Autodesk Fusion 360 part; units mm, degrees
sketch "Sketch1" plane through (0, 0, 0) normal (0, 0, 1) x (1, 0, 0)
  circle A0 centre (0, 0) radius 23.05
  line L0 (4.05, 4.05) -> (-4.05, 4.05) construction
  line L1 (-4.05, 4.05) -> (-4.05, -4.05) construction
  line L2 (-4.05, -4.05) -> (4.05, -4.05) construction
  line L3 (4.05, -4.05) -> (4.05, 4.05) construction
  line L4 (4.05, 4.05) -> (-4.05, -4.05) construction
  line L5 (-4.05, 4.05) -> (4.05, -4.05) construction
  circle A1 centre (0, 0) radius 1.95
  circle A2 centre (0, 0) radius 12
  line L6 (0, 0) -> (-9, -21.2203)
  line L7 (0, 0) -> (9, -21.2203)
  arc A3 (7.0767, -16.6855) -> (-7.0767, -16.6855) centre (0, -19.6868) ccw
  dimension "d1" = 46.1
  dimension "d2" = 8.1
  dimension "d3" = 8.1
  dimension "d4" = 3.9
  dimension "d5" = 24
  dimension "d19" = 18
  dimension "d20" = 9
extrude "Extrude1" add sketch "Sketch1" against normal blind 23.8
chamfer "Chamfer1" distance 11 distance2 5.8 1 edges at (-21.4901, -8.3352, 0) measured on face at (5.3767, -4.1064, 0)
extrude "Extrude2" add sketch "Sketch1" along normal blind 6.6 contours A1 L6 L7 | A1 L6 L7
chamfer "Chamfer2" distance 2 angle 45 1 edges at (-21.4901, 8.3352, -23.8)
hole "Hole1" at (-4.05, -4.05, 0) at (-4.05, 4.05, 0) at (4.05, 4.05, 0) at (4.05, -4.05, 0) direction (0, 0, -1) diameter 2.529 depth 5 tip angle 180
extrude "Extrude3" cut sketch "Sketch1" against normal up to surface (6.2 mm away) contours A0 L6 L7 A3
pattern_circular "C-Pattern1" count 4 over 360 about axis through (0, 0, 0) along (0, 0, 1) of "Extrude3"
equation "d9 = 23.8 mm - 18 mm"
equation "d20 = d19 / 2"
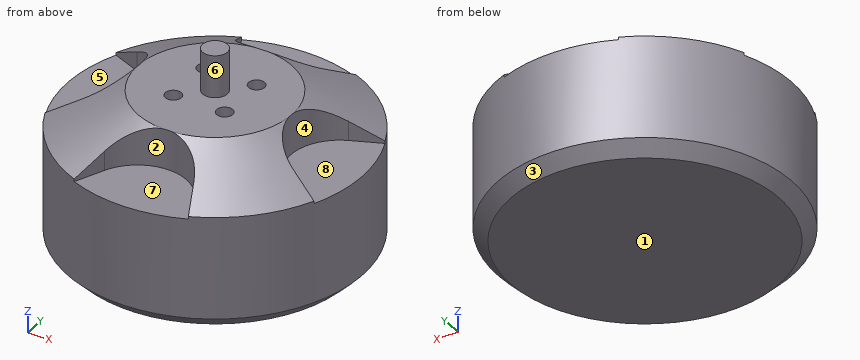
For this review, take the finished solid that the model builds, in its own axes (mm). Face numbers are marked on the shaded views. A direction names the side the tool comes from. Round coordinates to 2 decimals unless told otherwise and drop trailing zeros. Write each loop counter-clockwise with the first axis right and the second up, starting at its lowest first coordinate (ties: lowest second). Pieces come first, ordered by that corner, then holes. Notation, with made-up numbers: (70.25, -12.5) -> (129.25, -12.5) arc R10 ccw to (129.25, -4.5) -> close; hole circle Ø1 at (-29, -10). An arc over 180 degrees is marked (long way). One line per question, with ' | ' between items. Start each with the question number.
(1) Add section A-A, the plane x = 0. Write out the cut boundary in (y, z), plus the area to 3 significant figures.
(2) Add section B-B, the plane z = 4.5. Write out the cut boundary in (x, y).
(3) Mouldability with a two-part tool opening along Y and no side actions: class the marked faces 1, 2, 3 and 4 as released by +Y, released by -Y, zero draft, split by the parting line, or undercut.
(4) Tool access review of the marked faces 5, 6, 7 and 8: name each direction out of +Z, -Z, +X, -X, +Y, -Y from which nothing blocks a thin tool from reaching the whole face with its end or side.
(5) Insertion check: P1, Ø0.8, axis at x = 4.5, y = -4.5, coming from the +Z side; P2, Ø8, axis at x = 10, y = 15, coming from the +Z side; P3, Ø5.5, axis at x = 1.5, y = 16.5, coming from the +Z side. Each pin has a flat end and moves straight along its axis. Give the tip position at first contact, or say it passes through.
(6) For line 1 along Y through (x, z) = (-4.05, -3.2); line 2 along Y through (x, z) = (-5, -4); line 3 along X through (y, z) = (4.5, -4.5), list the stretches that pass through material, from the lowest coordinate up. Write a range as from..to.
Answer list:
1) outline: (-23.05, -21.8) -> (-21.05, -23.8) -> (21.05, -23.8) -> (23.05, -21.8) -> (23.05, -6.2) -> (12, -6.2) -> (12, 0) -> (1.95, 0) -> (1.95, 6.6) -> (-1.95, 6.6) -> (-1.95, 0) -> (-12, 0) -> (-12, -6.2) -> (-23.05, -6.2) -> close | area: 982 mm²
2) outline: circle Ø3.9 at (0, 0)
3) face 1: zero draft | face 2: released by -Y | face 3: split by the parting line | face 4: undercut
4) face 5: +Z, -X | face 6: +Z | face 7: +Z, -Y | face 8: +Z, +X
5) P1: z = -5 | P2: z = -1.04 | P3: z = -6.2
6) line 1: -13.15..-5.31, -2.79..2.79, 5.31..13.15 | line 2: -13.85..-4.88, -3.22..3.22, 4.88..13.85 | line 3: -13.45..-5.23, -2.87..2.87, 5.23..13.45
